Geometry check sheet. Reference: the model listing, model coordinates, mm. Coordinates: 2 decimals unless noted, no trailing zeros. Write each loop counter-clockwise with the first axis right and the second up, starting at its lowest first coordinate (ties: lowest second). Pieces come first, ordered by that corner, then holes. Notation, with made-up numbers: (39.5, 49) - (65.5, 49) arc R33 cw to (65.5, 82) - close; hole circle Ø5 at (50.25, -18). An arc over 180 degrees is marked (long way). Answer as a JSON object with one key per item and string values. Group by question number.
Autodesk Inventor part; units mm, degrees
ref_plane "YZ Plane" through (0, 0, 0) normal (1, 0, 0) x (0, 1, 0)
ref_plane "XZ Plane" through (0, 0, 0) normal (0, 1, 0) x (-1, 0, 0)
ref_plane "XY Plane" through (0, 0, 0) normal (0, 0, 1) x (1, 0, 0)
sketch "Boceto1" plane through (0, 0, 0) normal (0, 1, 0) x (-1, 0, 0)
  line L0 (-192, 193.5) -> (192, -193.5) construction
  line L1 (192, 193.5) -> (-192, -193.5) construction
  line L2 (-192, -168.5) -> (-195, -168.5)
  line L3 (-195, -168.5) -> (-195, -68.5)
  line L4 (-195, -68.5) -> (-192, -68.5)
  line L5 (-192, -193.5) -> (-192, -168.5)
  line L6 (-192, -18.5) -> (-195, -18.5)
  line L7 (-195, -18.5) -> (-195, 81.5)
  line L8 (-195, 81.5) -> (-192, 81.5)
  line L9 (-192, -68.5) -> (-192, -18.5)
  line L10 (-192, 81.5) -> (-192, 193.5)
  line L11 (100, 93.5) -> (50, 93.5)
  line L12 (50, 93.5) -> (50, 96.5)
  line L13 (50, 96.5) -> (100, 96.5)
  line L14 (100, 96.5) -> (100, 93.5)
  line L15 (-50, 96.5) -> (-100, 96.5)
  line L16 (-100, 96.5) -> (-100, 93.5)
  line L17 (-100, 93.5) -> (-50, 93.5)
  line L18 (-50, 93.5) -> (-50, 96.5)
  line L19 (-125, -193.5) -> (-125, -196.5)
  line L20 (-125, -196.5) -> (-25, -196.5)
  line L21 (-25, -196.5) -> (-25, -193.5)
  line L22 (25, -193.5) -> (25, -196.5)
  line L23 (25, -196.5) -> (125, -196.5)
  line L24 (125, -196.5) -> (125, -193.5)
  line L25 (-125, -193.5) -> (-192, -193.5)
  line L26 (192, -193.5) -> (125, -193.5)
  line L27 (25, -193.5) -> (-25, -193.5)
  line L28 (-192, 193.5) -> (192, 193.5)
  line L29 (192, -168.5) -> (195, -168.5)
  line L30 (195, -168.5) -> (195, -68.5)
  line L31 (195, -68.5) -> (192, -68.5)
  line L32 (192, -18.5) -> (195, -18.5)
  line L33 (195, -18.5) -> (195, 81.5)
  line L34 (195, 81.5) -> (192, 81.5)
  line L35 (192, -168.5) -> (192, -193.5)
  line L36 (192, 193.5) -> (192, 81.5)
  line L37 (192, -18.5) -> (192, -68.5)
  point P0 (0, 0)
  dimension "d5" = 100
  dimension "d7" = 100
  dimension "d8" = 50
  dimension "d9" = 3
  dimension "d12" = 50
  dimension "d13" = 3
  dimension "d14" = 100
  dimension "d59" = 100
  dimension "d61" = 100
  dimension "d63" = 50
  dimension "d64" = 3
  dimension "d75" = 25
  dimension "d76" = 50
  dimension "d77" = 100
  dimension "d78" = 3
  dimension "d79" = 3
  dimension "d81" = 3
  dimension "d83" = 390
  dimension "d84" = 390
  dimension "d85" = 67
extrude "Extrusión2" add sketch "Boceto1" along normal blind 3
sketch "Boceto2" plane through (0, 3, 0) normal (0, 1, 0) x (1, 0, 0)
  line L0 (72, -93.5) -> (72, 193.5) construction
  line L1 (192, 193.5) -> (-192, 193.5)
  line L2 (50, -93.5) -> (100, -93.5)
  line L3 (72, 50) -> (192, 50) construction
  line L4 (192, 18.5) -> (192, 68.5)
  line L5 (117, 153) -> (167, 153)
  line L6 (167, 153) -> (167, 150)
  line L7 (167, 150) -> (117, 150)
  line L8 (117, 150) -> (117, 153)
  line L9 (117, -50) -> (167, -50)
  line L10 (167, -50) -> (167, -53)
  line L11 (167, -53) -> (117, -53)
  line L12 (117, -53) -> (117, -50)
  line L13 (89, 100) -> (92, 100)
  line L14 (92, 100) -> (92, 0)
  line L15 (92, 0) -> (89, 0)
  line L16 (89, 0) -> (89, 100)
  point P0 (0, 0)
  point P1 (92, 50)
  dimension "d18" = 120
  dimension "d19" = 50
  dimension "d20" = 3
  dimension "d21" = 50
  dimension "d22" = 3
  dimension "d23" = 100
  dimension "d24" = 100
  dimension "d25" = 25
  dimension "d26" = 3
  dimension "d27" = 100
  dimension "d28" = 28
extrude "Extrusión3" cut sketch "Boceto2" against normal blind 3
hole "Agujero1" at (92, 3, -168.5) direction (0, -1, 0) diameter 5 end through all
hole "Agujero2" at (-92, 3, -168.5) direction (0, -1, 0) diameter 5 end through all
sketch "Boceto3" plane through (0, 3, 0) normal (0, 1, 0) x (1, 0, 0)
  circle A0 centre (92, -68.5) radius 2.5
  circle A1 centre (-92, -68.5) radius 2.5
  line L0 (-192, 193.5) -> (-192, -193.5)
  line L1 (192, -193.5) -> (192, -81.5)
  line L2 (-100, -93.5) -> (-50, -93.5)
  line L3 (99.5, -70) -> (96.5, -70)
  line L4 (96.5, -70) -> (96.5, -67)
  line L5 (96.5, -67) -> (99.5, -67)
  line L6 (99.5, -67) -> (99.5, -70)
  line L7 (-96.5, -70) -> (-99.5, -70)
  line L8 (-99.5, -70) -> (-99.5, -67)
  line L9 (-99.5, -67) -> (-96.5, -67)
  line L10 (-96.5, -67) -> (-96.5, -70)
  point P0 (0, 0)
  point P1 (99.5, -68.5)
  point P2 (-96.5, -68.5)
  dimension "d49" = 5
  dimension "d50" = 5
  dimension "d51" = 100
  dimension "d52" = 25
  dimension "d54" = 100
  dimension "d98" = 3
  dimension "d99" = 3
  dimension "d101" = 4.5
  dimension "d102" = 3
  dimension "d103" = 3
  dimension "d105" = 4.5
extrude "Extrusión4" cut sketch "Boceto3" against normal blind 3
sketch "Boceto4" plane through (0, 3, 0) normal (0, 1, 0) x (1, 0, 0)
  line L0 (-127, 150.5) -> (-157, 150.5)
  line L1 (-157, 150.5) -> (-157, 147.5)
  line L2 (-157, 147.5) -> (-127, 147.5)
  line L3 (-127, 147.5) -> (-127, 150.5)
  line L4 (-192, 193.5) -> (-192, 168.5)
  line L5 (-127, -46.5) -> (-157, -46.5)
  line L6 (-157, -46.5) -> (-157, -49.5)
  line L7 (-157, -49.5) -> (-127, -49.5)
  line L8 (-127, -49.5) -> (-127, -46.5)
  line L9 (-125, 193.5) -> (-192, 193.5)
  line L10 (-139.5, 152.5) -> (-144.5, 152.5)
  line L11 (-144.5, 152.5) -> (-144.5, 155.5)
  line L12 (-144.5, 155.5) -> (-139.5, 155.5)
  line L13 (-139.5, 155.5) -> (-139.5, 152.5)
  point P0 (0, 0)
  point P1 (-142, 152.5)
  point P2 (-142, 150.5)
  dimension "d86" = 30
  dimension "d87" = 3
  dimension "d88" = 35
  dimension "d89" = 30
  dimension "d90" = 3
  dimension "d93" = 194
  dimension "d94" = 43
  dimension "d95" = 5
  dimension "d96" = 3
  dimension "d97" = 2
extrude "Extrusión5" cut sketch "Boceto4" against normal blind 3 contours L3 L2 L1 L0 | L10 L11 L12 L13
properties part number "Base"
(1) Section check B-B (z = -29). Record the cut outline in (x, y).
(2) Section check A-A (x = 143). Record the cut outline in (y, z).
(3) Section check C-C (y = 1.15). Count the separate pieces of the cut face and the enclosed holes in it, and give its area (3 significant figures).
(4) Gauge pin test, flat ends, axial feed: pin 1 (5 mm diameter, centred on x = -60.5, z = -37.5, fed in from -Y); pin 2 (0.9 mm diameter, centred on y = 2, z = 95.5, fed in from +X); pin 3 (0.9 mm diameter, centred on x = -141.5, y = 1.5, fed in from -Z); pin 4 (4.5 mm diameter, centred on x = 92, z = -168.5, fed in from +Y). Record the tip position at first contact, or that the pin passes through.
(5) Material ranges on L1, parallel to X at y = 2, z = 68.5; L2, parallel to Z at x = -92, y = 1.05; L3, parallel to Z at x = 146, y = 0.4, recorded low to high. Write a range as [from, to].
Conclusion:
{
 "1": {"outline": "(-192, 0) - (89, 0) - (89, 3) - (-192, 3) - close; (92, 0) - (192, 0) - (192, 3) - (92, 3) - close"},
 "2": {"outline": "(0, -193.5) - (3, -193.5) - (3, -153) - (0, -153) - close; (0, -150) - (3, -150) - (3, 50) - (0, 50) - close; (0, 53) - (3, 53) - (3, 193.5) - (0, 193.5) - close"},
 "3": {"separate pieces": "1", "enclosed holes": "13", "area": "149,000 mm^2"},
 "4": {"pin 1": "stops at y = 0", "pin 2": "stops at x = 192", "pin 3": "stops at z = -193.5", "pin 4": "passes through"},
 "5": {"L1": "x = [-195, -99.5], [-96.5, -94.5], [-89.5, 89.5], [94.5, 96.5], [99.5, 195]", "L2": "z = [-196.5, -171], [-166, 66], [71, 93.5], [96.5, 193.5]", "L3": "z = [-193.5, -153], [-150, 50], [53, 193.5]"}
}
